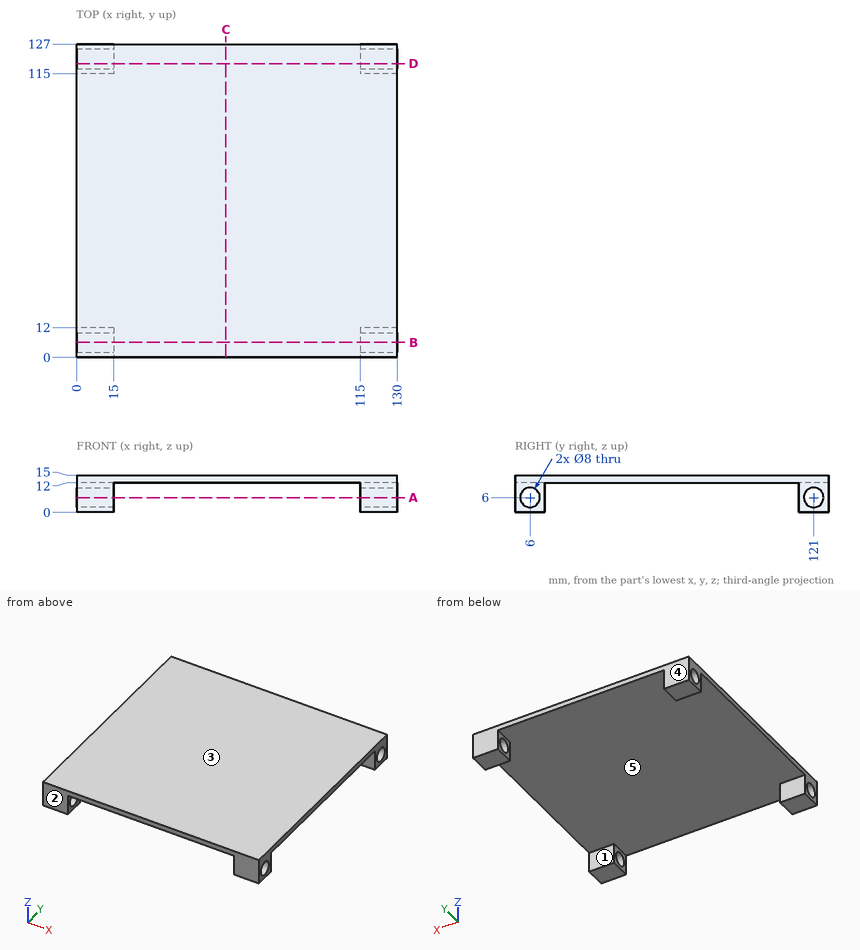
The figure shows three views and two pictorial views of one solid part (mm, origin at its lowest corner). Answer the questions. A direction names the side the tool comes from. Round coordinates to 2 decimals unless told otherwise and drop trailing zeros. Write each loop counter-clockwise with the first axis right and the second up, starting at its lowest first coordinate (ties: lowest second). Pieces come first, ordered by that corner, then holes. Notation, with made-up numbers: M 25,34.5 L 29,34.5 A20 cw 29,57.5 Z; hole C -15,-5.75 d7. An arc over 180 degrees is marked long. Write each question's results on one line, items separated by ' | '. Start each with the question number.
(1) Find the intervals of material crossed by line 1 (Y direction, x = 122, z = 6); line 2 (X direction, y = 11, z = 5); line 3 (Z direction, x = 15, y = 15.5), in increasing order.
(2) The part is cut by section D-D, the plane y = 119. Write down the section's boundary in (x, z).
(3) For the marked faces 1 and 2, determine the directions among +Z, -Z, +X, -X, +Y, -Y from which every point of the face is accessible in a straight line to the end or side of a thin tool.
(4) Determine the mould class of the marked faces 3, 4 and 5 for opening direction Y: +Y half, -Y half, draft (parallel to the pull), parting line (faces both ways), or undercut.
(5) Each of these flat-tipped pins is pushed along its axis until it touches: P1, Ø8, axis at x = 84.5, z = 5.5, coming from the -Y side; P2, Ø8, axis at x = 22.5, y = 14.5, coming from the -Z side. Where does it stop, or does it pass through?
(6) The part is cut by section C-C, the plane x = 60.5. Write down the section's boundary in (y, z).
(7) The part is cut by section B-B, the plane y = 6. Write down the section's boundary in (x, z).
(8) The part is cut by section A-A, the plane z = 6. Give the number of separate pieces and of enclosed holes in the cut face, and give its area (3 significant figures).
Worked answers:
1) line 1: y = 0 to 2, 10 to 12, 115 to 117, 125 to 127 | line 2: x = 0 to 15, 115 to 130 | line 3: z = 12 to 15
2) outline: M 0,0 L 15,0 L 15,2.54 L 0,2.54 Z; M 0,9.46 L 15,9.46 L 15,12 L 115,12 L 115,9.46 L 130,9.46 L 130,15 L 0,15 Z; M 115,0 L 130,0 L 130,2.54 L 115,2.54 Z
3) face 1: -Z, +X, -X | face 2: +Z, -Z, +X, -X, -Y
4) face 3: draft | face 4: +Y half | face 5: undercut
5) P1: passes through | P2: stops at z = 12
6) outline: M 0,12 L 127,12 L 127,15 L 0,15 Z
7) outline: M 0,0 L 15,0 L 15,2 L 0,2 Z; M 0,10 L 15,10 L 15,12 L 115,12 L 115,10 L 130,10 L 130,15 L 0,15 Z; M 115,0 L 130,0 L 130,2 L 115,2 Z
8) separate pieces: 8 | enclosed holes: 0 | area: 240 mm²
